Could you check a few things on this model? Use its own coordinates, in mm. A direction names the side the tool comes from. Coordinates: 2 decimals unless noted, no trailing zeros. Loops run counter-clockwise (first coordinate to the right, second up) from the corner with the lowest first, then second, coordinate; pieces in that order, holes last.
from build123d import *

# Parameters (mm, degrees)
SKETCH_W         = 65.5
SKETCH_H         = 65.5
PAD_DEPTH        = 10
SKETCH001_R      = 3.55
SKETCH001_R_2    = 2.5
PAD001_DEPTH     = 3
SKETCH002_R      = 2
POCKET_DEPTH     = 8
CHAMFER_SIZE     = 0.2
POCKET001_DEPTH  = 2.5
SKETCH004_W      = 40.5
SKETCH004_H      = 3.5
POCKET002_DEPTH  = 2
SKETCH005_W      = 40.5
SKETCH005_H      = 3.5
POCKET003_DEPTH  = 2
SKETCH006_W      = 65.5
SKETCH006_H      = 7.15
POCKET004_DEPTH  = 4
SKETCH007_W      = 65.5
SKETCH007_H      = 7.15
POCKET005_DEPTH  = 4
SKETCH008_R      = 0.925
POCKET006_DEPTH  = 2.15
CHAMFER001_SIZE2 = 0.25
CHAMFER001_SIZE  = 1
SKETCH009_R      = 5.25
POCKET007_DEPTH  = 1.25


with BuildPart() as part:
    # Sketch → Pad (new body)
    with BuildSketch(Plane.XY):
        Rectangle(SKETCH_W, SKETCH_H)
    extrude(amount=PAD_DEPTH)

    # Sketch001 (on Face6 of Pad) → Pad001 (join)
    with BuildSketch(Plane.XY.offset(10)):
        with Locations((0, 19.85)):
            Circle(SKETCH001_R)
        with Locations((0, -19.85)):
            Circle(SKETCH001_R_2)
    extrude(amount=PAD001_DEPTH)

    # Sketch002 (on Face10 of Pad001) → Pocket (cut)
    with BuildSketch(Plane.XY.offset(13)):
        with Locations((0, 19.85)):
            Circle(SKETCH002_R)
        with Locations((0, -19.85)):
            Circle(SKETCH002_R)
    extrude(amount=-POCKET_DEPTH, mode=Mode.SUBTRACT)

    # Chamfer
    chamfer_edges = [part.edges().sort_by_distance(p)[0] for p in [
        (-3.55, 19.85, 13),
        (-2.5, -19.85, 13),
    ]]
    chamfer(chamfer_edges, length=CHAMFER_SIZE)

    # Sketch003 (on DatumPlane) → Pocket001 (cut)
    with BuildSketch(Plane.XY.offset(5)):
        Polygon((-3.650297, 17.7425), (0, 15.635), (3.650297, 17.7425), (3.650297, 21.9575), (0, 24.065), (-3.650297, 21.9575), align=None)
        Polygon((-3.650297, -21.9575), (0, -24.065), (3.650297, -21.9575), (3.650297, -17.7425), (0, -15.635), (-3.650297, -17.7425), align=None)
    extrude(amount=-POCKET001_DEPTH, mode=Mode.SUBTRACT)

    # Sketch004 (on Face7 of Pocket001) → Pocket002 (cut)
    with BuildSketch(Plane.YZ.offset(32.75)):
        with Locations((0, 5)):
            Rectangle(SKETCH004_W, SKETCH004_H)
    extrude(amount=-POCKET002_DEPTH, mode=Mode.SUBTRACT)

    # Sketch005 (on Face6 of Pocket002) → Pocket003 (cut)
    with BuildSketch(Plane(origin=(-32.75, 0, 0), x_dir=(0, -1, 0), z_dir=(-1, 0, 0))):
        with Locations((0, 5)):
            Rectangle(SKETCH005_W, SKETCH005_H)
    extrude(amount=-POCKET003_DEPTH, mode=Mode.SUBTRACT)

    # Sketch006 (on DatumPlane) → Pocket004 (cut)
    with BuildSketch(Plane.YZ.offset(30.75)):
        with Locations((0, 5)):
            Rectangle(SKETCH006_W, SKETCH006_H)
    extrude(amount=-POCKET004_DEPTH, mode=Mode.SUBTRACT)

    # Sketch007 (on DatumPlane) → Pocket005 (cut)
    with BuildSketch(Plane(origin=(-30.75, 0, 0), x_dir=(0, -1, 0), z_dir=(-1, 0, 0))):
        with Locations((0, 5)):
            Rectangle(SKETCH007_W, SKETCH007_H)
    extrude(amount=-POCKET005_DEPTH, mode=Mode.SUBTRACT)

    # Sketch008 (on Face11 of Pocket005) → Pocket006 (cut)
    with BuildSketch(Plane(origin=(0, 0, 0), x_dir=(1, 0, 0), z_dir=(0, 0, -1))):
        with Locations((-25, 25)):
            Circle(SKETCH008_R)
        with Locations((25, 25)):
            Circle(SKETCH008_R)
        with Locations((-25, -25)):
            Circle(SKETCH008_R)
        with Locations((25, -25)):
            Circle(SKETCH008_R)
    extrude(amount=-POCKET006_DEPTH, mode=Mode.SUBTRACT)

    # Chamfer001
    chamfer001_edges = [part.edges().sort_by_distance(p)[0] for p in [
        (-25.925, -25, 0),
        (24.075, -25, 0),
        (-25.925, 25, 0),
        (24.075, 25, 0),
    ]]
    chamfer001_side = part.faces().sort_by_distance((0, 0, 0))[0]
    chamfer(chamfer001_edges, length=CHAMFER001_SIZE, length2=CHAMFER001_SIZE2, reference=chamfer001_side)

    # Sketch009 (on Face11 of Chamfer001) → Pocket007 (cut)
    with BuildSketch(Plane.XY.offset(10)):
        with Locations((-20, 19.85)):
            Circle(SKETCH009_R)
        with Locations((20, 19.85)):
            Circle(SKETCH009_R)
        with Locations((20, -19.85)):
            Circle(SKETCH009_R)
        with Locations((-20, -19.85)):
            Circle(SKETCH009_R)
    extrude(amount=-POCKET007_DEPTH, mode=Mode.SUBTRACT)


solid = part.part
1) We'd pull the mould along X, two halves only. Please class faces 1 (the flat face through (-25, -25, 2.15)), 2 (the flat face through (-32, 0, 3.25)), 3 (the cylindrical face through (1.34, -17.74, 11.38)): released by +X, released by -X, zero draft, split by the parting line, or undercut.
2) Imagine slicing it at B-B on x = -15.5. List the corners of the cut face in (y, z) for me, plus the area to 3 significant figures.
3) If I drill on L1, parallel to X at y = -25, z = 1.6 (3 decimals); L2, parallel to Y at x = -25, z = 0.95 (3 decimals), over which ranges is the centre line in solid material (lowest first)?
4) Will these pins go through, and if not, where does the flat tip stop? pin 1 (12 mm diameter, centred on x = -20, y = -19.85, fed in from +Z); pin 2 (0.6 mm diameter, centred on x = 24.5, y = -24.5, fed in from -Z); pin 3 (1.5 mm diameter, centred on x = 25, y = 25, fed in from -Z).
5) Imagine slicing it at C-C on x = 22. List the corners of the cut face in (y, z) for me, plus the area to 3 significant figures.
6) For faces 4 (the flat face through (-1.8, 23.026, 3.768)), 5 (the flat face through (32, 0, 3.25)), 6 (the flat face through (26.75, 0, 5)), which set-ups out of +Z, -Z, +X, -X, +Y, -Y let a thin tool reach every point of the face, with its end or its side?
7) Imagine slicing it at A-A on y = 11.5. List the corners of the cut face in (x, z) for me (3 decimals), plus the area to 3 significant figures.
Solved:
1. face 1: undercut
1. face 2: zero draft
1. face 3: split by the parting line
2. outline: (-32.75, 0) - (32.75, 0) - (32.75, 10) - (22.55, 10) - (22.55, 8.75) - (17.15, 8.75) - (17.15, 10) - (-17.15, 10) - (-17.15, 8.75) - (-22.55, 8.75) - (-22.55, 10) - (-32.75, 10) - close
2. area: 641 mm2
3. L1: x = -32.75 to -30.75, -26.75 to -25.925, -24.075 to 24.075, 25.925 to 26.75, 30.75 to 32.75
3. L2: y = -32.75 to -25.925, -24.075 to 24.075, 25.925 to 32.75
4. pin 1: stops at z = 10
4. pin 2: stops at z = 0.23
4. pin 3: stops at z = 2.15
5. outline: (-32.75, 0) - (32.75, 0) - (32.75, 10) - (24.7, 10) - (24.7, 8.75) - (15, 8.75) - (15, 10) - (-15, 10) - (-15, 8.75) - (-24.7, 8.75) - (-24.7, 10) - (-32.75, 10) - close
5. area: 631 mm2
6. face 4: none
6. face 5: +X
6. face 6: +Y, -Y
7. outline: (-32.75, 0) - (32.75, 0) - (32.75, 3.25) - (30.75, 3.25) - (30.75, 1.425) - (26.75, 1.425) - (26.75, 8.575) - (30.75, 8.575) - (30.75, 6.75) - (32.75, 6.75) - (32.75, 10) - (-32.75, 10) - (-32.75, 6.75) - (-30.75, 6.75) - (-30.75, 8.575) - (-26.75, 8.575) - (-26.75, 1.425) - (-30.75, 1.425) - (-30.75, 3.25) - (-32.75, 3.25) - close
7. area: 584 mm2
